from build123d import *

# Parameters (mm, degrees)
SKETCH1_W            = 20
SKETCH1_H            = 20
BOSS_EXTRUDE1_DEPTH  = 20
SKETCH2_W            = 45
SKETCH2_H            = 70
BOSS_EXTRUDE2_DEPTH  = 12
CUT_EXTRUDE1_DEPTH   = 5.8
FILLET1_R            = 3.6
FILLET2_R            = 10
SKETCH5_R            = 3.9
CUT_EXTRUDE2_DEPTH   = 53.490475326
CUT_EXTRUDE3_REACH   = 51.17
SKETCH6_R            = 1.75
SKETCH7_W            = 12
SKETCH7_H            = 45
CUT_EXTRUDE4_DEPTH   = 4.8
SKETCH9_W            = 12
SKETCH9_H            = 45
CUT_EXTRUDE5_DEPTH   = 23.8
SKETCH10_W           = 12.5
SKETCH10_H           = 41.4
CUT_EXTRUDE6_DEPTH   = 23.8
SKETCH11_W           = 20
SKETCH11_H           = 1.2
CUT_EXTRUDE7_DEPTH   = 23.8
BOSS_EXTRUDE3_START  = 20
SKETCH12_W           = 20
SKETCH12_H           = 20
SKETCH12_R           = 3.9
BOSS_EXTRUDE3_DEPTH  = 20
SKETCH13_W           = 20.2
SKETCH13_H           = 20.2
SKETCH13_R           = 3.9
BOSS_EXTRUDE4_DEPTH  = 40
SKETCH14_W           = 12
SKETCH14_H           = 20
BOSS_EXTRUDE5_DEPTH  = 0.1
SKETCH17_R           = 4.83091966
BOSS_EXTRUDE8_DEPTH  = 39
SKETCH18_W           = 20.2
SKETCH18_H           = 20.2
CUT_EXTRUDE8_DEPTH   = 40
FILLET4_R            = 4
SKETCH20_W           = 12
SKETCH20_H           = 20
BOSS_EXTRUDE9_DEPTH  = 8
SKETCH21_W           = 47.2
SKETCH21_H           = 20
BOSS_EXTRUDE11_DEPTH = 10
SKETCH23_W           = 20
SKETCH23_H           = 20
BOSS_EXTRUDE12_DEPTH = 30
SKETCH25_W           = 20
SKETCH25_H           = 40.2
BOSS_EXTRUDE13_DEPTH = 57.5
SKETCH26_W           = 20
SKETCH26_H           = 20.8
CUT_EXTRUDE9_DEPTH   = 40.9
SKETCH27_R           = 2.35
CUT_EXTRUDE10_DEPTH  = 10
SKETCH28_R           = 2.35
CUT_EXTRUDE11_DEPTH  = 140.85113514
CHAMFER1_SIZE        = 1
FILLET5_R            = 7


with BuildPart() as part:
    # Sketch1 → Boss-Extrude1 (new body)
    with BuildSketch(Plane(origin=(0, 0, 0), x_dir=(0, 0, -1), z_dir=(1, 0, 0))):
        Rectangle(SKETCH1_W, SKETCH1_H)
    extrude(amount=BOSS_EXTRUDE1_DEPTH)

    # Sketch2 → Boss-Extrude2 (add)
    with BuildSketch(Plane(origin=(20, 0, 0), x_dir=(0, 0, -1), z_dir=(1, 0, 0))):
        Rectangle(SKETCH2_W, SKETCH2_H)
    extrude(amount=BOSS_EXTRUDE2_DEPTH)

    # Sketch4 → Cut-Extrude1 (cut)
    with BuildSketch(Plane(origin=(32, 0, 0), x_dir=(0, 0, -1), z_dir=(1, 0, 0))):
        with BuildLine():
            Line((3.6, -28.55), (-3.6, -28.55))
            Line((-3.6, -28.55), (-3.6, -7.311805523))
            ThreePointArc((-3.6, -7.311805523), (0, 8.15), (3.6, -7.311805523))
            Line((3.6, -7.311805523), (3.6, -28.55))
        make_face()
    extrude(amount=-CUT_EXTRUDE1_DEPTH, mode=Mode.SUBTRACT)

    # Fillet1
    fillet1_edges = [part.edges().sort_by_distance(p)[0] for p in [
        (29.1, -28.55, 3.6),
        (29.1, -28.55, -3.6),
    ]]
    fillet(fillet1_edges, radius=FILLET1_R - 0.0001)  # a hair under: the kernel refuses the full size

    # Fillet2
    fillet2_edges = [part.edges().sort_by_distance(p)[0] for p in [
        (29.1, -7.311805523, 3.6),
        (29.1, -7.311805523, -3.6),
    ]]
    fillet(fillet2_edges, radius=FILLET2_R)

    # Sketch5 → Cut-Extrude2 (cut, through all)
    with BuildSketch(Plane.ZY):
        Circle(SKETCH5_R)
    extrude(amount=-CUT_EXTRUDE2_DEPTH, mode=Mode.SUBTRACT)

    # Sketch6 → Cut-Extrude3 (cut, up to next)
    with BuildSketch(Plane(origin=(26.2, 0, 0), x_dir=(0, 0, -1), z_dir=(1, 0, 0)), mode=Mode.PRIVATE) as cut_extrude3_sk1:
        with Locations((0, -20.6)):
            Circle(SKETCH6_R)
    cut_extrude3_tool1 = extrude(cut_extrude3_sk1.sketch, amount=-CUT_EXTRUDE3_REACH, mode=Mode.PRIVATE) & part.part
    # Sketch6 → Cut-Extrude3 (cut, up to next)
    with BuildSketch(Plane(origin=(26.2, 0, 0), x_dir=(0, 0, -1), z_dir=(1, 0, 0)), mode=Mode.PRIVATE) as cut_extrude3_sk2:
        with Locations((0, -9.35)):
            Circle(SKETCH6_R)
    cut_extrude3_tool2 = extrude(cut_extrude3_sk2.sketch, amount=-CUT_EXTRUDE3_REACH, mode=Mode.PRIVATE) & part.part
    add(cut_extrude3_tool1.solids().sort_by_distance((26.2, -20.6, 0))[0], mode=Mode.SUBTRACT)
    add(cut_extrude3_tool2.solids().sort_by_distance((26.2, -9.35, 0))[0], mode=Mode.SUBTRACT)

    # Sketch7 → Cut-Extrude4 (cut)
    with BuildSketch(Plane.XZ.offset(35)):
        with Locations((26, 0)):
            Rectangle(SKETCH7_W, SKETCH7_H)
    extrude(amount=-CUT_EXTRUDE4_DEPTH, mode=Mode.SUBTRACT)

    # Sketch9 → Cut-Extrude5 (cut)
    with BuildSketch(Plane(origin=(0, 35, 0), x_dir=(1, 0, 0), z_dir=(0, 1, 0))):
        with Locations((26, 0)):
            Rectangle(SKETCH9_W, SKETCH9_H)
    extrude(amount=-CUT_EXTRUDE5_DEPTH, mode=Mode.SUBTRACT)

    # Sketch10 → Cut-Extrude6 (cut)
    with BuildSketch(Plane.ZY.offset(-20)):
        with Locations((-16.25, -9.5)):
            Rectangle(SKETCH10_W, SKETCH10_H)
        with Locations((16.25, -9.5)):
            Rectangle(SKETCH10_W, SKETCH10_H)
    extrude(amount=-CUT_EXTRUDE6_DEPTH, mode=Mode.SUBTRACT)

    # Sketch11 → Cut-Extrude7 (cut)
    with BuildSketch(Plane.ZY.offset(-20)):
        with Locations((0, 10.6)):
            Rectangle(SKETCH11_W, SKETCH11_H)
    extrude(amount=-CUT_EXTRUDE7_DEPTH, mode=Mode.SUBTRACT)

    # Sketch12 → Boss-Extrude3 (add)
    with BuildSketch(Plane.ZY.offset(BOSS_EXTRUDE3_START)):
        Rectangle(SKETCH12_W, SKETCH12_H)
        Circle(SKETCH12_R, mode=Mode.SUBTRACT)
    extrude(amount=-BOSS_EXTRUDE3_DEPTH)

    # Sketch13 → Boss-Extrude4 (add)
    with BuildSketch(Plane.ZY.offset(20)):
        Rectangle(SKETCH13_W, SKETCH13_H)
        Circle(SKETCH13_R, mode=Mode.SUBTRACT)
    extrude(amount=-BOSS_EXTRUDE4_DEPTH)

    # Sketch14 → Boss-Extrude5 (add)
    with BuildSketch(Plane(origin=(0, 10, 0), x_dir=(1, 0, 0), z_dir=(0, 1, 0))):
        with Locations((26, 0)):
            Rectangle(SKETCH14_W, SKETCH14_H)
    extrude(amount=BOSS_EXTRUDE5_DEPTH)

    # Sketch17 → Boss-Extrude8 (add)
    with BuildSketch(Plane.ZY.offset(20)):
        Circle(SKETCH17_R)
    extrude(amount=-BOSS_EXTRUDE8_DEPTH)

    # Sketch18 → Cut-Extrude8 (cut)
    with BuildSketch(Plane.ZY.offset(20)):
        Rectangle(SKETCH18_W, SKETCH18_H)
    extrude(amount=-CUT_EXTRUDE8_DEPTH, mode=Mode.SUBTRACT)

    # Fillet4
    fillet4_edges = [part.edges().sort_by_distance(p)[0] for p in [
        (26, 10.1, -10),
        (26, 10.1, 10),
    ]]
    fillet(fillet4_edges, radius=FILLET4_R)

    # Sketch20 → Boss-Extrude9 (add)
    with BuildSketch(Plane.XZ.offset(30.2)):
        with Locations((26, 0)):
            Rectangle(SKETCH20_W, SKETCH20_H)
    extrude(amount=BOSS_EXTRUDE9_DEPTH)

    # Sketch21 → Boss-Extrude11 (add)
    with BuildSketch(Plane.XZ.offset(38.2)):
        with Locations((43.6, 0)):
            Rectangle(SKETCH21_W, SKETCH21_H)
    extrude(amount=BOSS_EXTRUDE11_DEPTH)

    # Sketch23 → Boss-Extrude12 (add)
    with BuildSketch(Plane.XZ.offset(48.2)):
        with Locations((57.2, 0)):
            Rectangle(SKETCH23_W, SKETCH23_H)
    extrude(amount=BOSS_EXTRUDE12_DEPTH)

    # Sketch25 → Boss-Extrude13 (add)
    with BuildSketch(Plane.XZ.offset(78.2)):
        with Locations((57.2, 0)):
            Rectangle(SKETCH25_W, SKETCH25_H)
    extrude(amount=BOSS_EXTRUDE13_DEPTH)

    # Sketch26 → Cut-Extrude9 (cut)
    with BuildSketch(Plane.XZ.offset(135.7)):
        with Locations((57.2, 0)):
            Rectangle(SKETCH26_W, SKETCH26_H)
    extrude(amount=-CUT_EXTRUDE9_DEPTH, mode=Mode.SUBTRACT)

    # Sketch27 → Cut-Extrude10 (cut)
    with BuildSketch(Plane(origin=(0, -135.7, 0), x_dir=(-1, 0, 0), z_dir=(0, -1, 0))):
        with Locations(Location((-57.2, 15.25, 0), (0, 0, 90))):
            Circle(SKETCH27_R)
        with Locations(Location((-57.2, -15.25, 0), (0, 0, 270))):
            Circle(SKETCH27_R)
    extrude(amount=-CUT_EXTRUDE10_DEPTH, mode=Mode.SUBTRACT)

    # Sketch28 → Cut-Extrude11 (cut, through all)
    with BuildSketch(Plane.ZY.offset(-47.2)):
        with Locations((4.9, -90.91)):
            Circle(SKETCH28_R)
        with Locations(Location((-4.9, -90.91, 0), (0, 0, 180))):
            Circle(SKETCH28_R)
    extrude(amount=-CUT_EXTRUDE11_DEPTH, mode=Mode.SUBTRACT)

    # Chamfer1
    chamfer1_edges = [part.edges().sort_by_distance(p)[0] for p in [
        (57.2, -135.7, -12.9),
        (57.2, -135.7, 12.9),
        (47.2, -90.91, 2.55),
        (47.2, -90.91, -2.55),
    ]]
    chamfer(chamfer1_edges, length=CHAMFER1_SIZE)

    # Fillet5
    fillet5_edges = [part.edges().sort_by_distance(p)[0] for p in [
        (32, -38.2, 0),
        (47.2, -48.2, 0),
    ]]
    fillet(fillet5_edges, radius=FILLET5_R)


solid = part.part
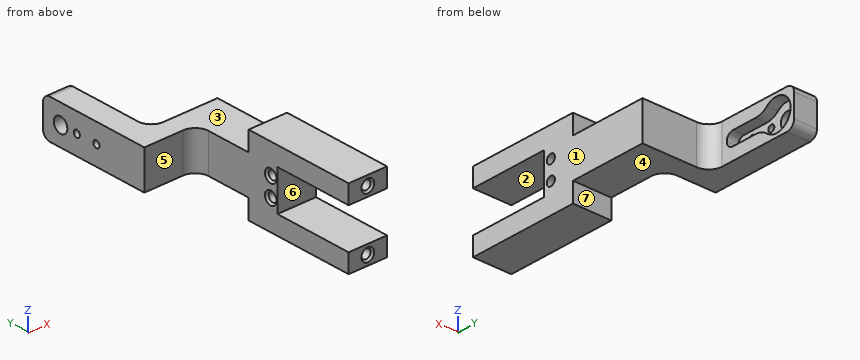
The model under review builds one solid part; all positions refer to its coordinate system, in mm. Face numbers are marked on the shaded views. A direction names the side the tool comes from. Give positions to 0.01 mm unless a question says otherwise; leave off trailing zeros. Order: outer loops, then holes, each group sorted by start corner. A loop starts at its lowest first (then second) coordinate and runs counter-clockwise, first axis right, second up. Notation, with made-up numbers: M 43.5,65 L 84.5,65 A16 ccw 84.5,95 Z; hole C -20,86.25 d2. An arc over 180 degrees is marked long. Use one line per item in the form item = value. Start each with the question number.
Item 1: To check wall thickness, follow line 1 along Y through (x, z) = (21.75, 0); line 2 along Y through (x, z) = (27.8, 0); line 3 along Z through (x, y) = (55.5, -92.5). State the ranges of each line that lie inside material, in increasing order. Write a range as from..to.
Item 2: We need section C-C on y = -15. Give the boundary of the cut face in (x, z), plus the area to 3 significant figures.
Item 3: For the marked faces 5, 6 and 7, list the 3-axis set-ups (+Z, -Z, +X, -X, +Y, -Y) from which the entire face can be reached by the end or side of a thin tool; tool diameter is ignored.
Item 4: We need section B-B on z = 15.25. Give the boundary of the cut face in (x, y).
Item 5: The part is to be moulded in two halves that separate along Z. For the marked faces 1, 2, 3 and 4, say which applies: pulls with the +Z half, pulls with the -Z half, needs draft (parallel to the pull), parting line crosses it, or undercut.
Item 6: Insertion check: pin 1 Ø10 at (x, z) = (31.5, 2) entering from -Y; pin 2 Ø2 at (y, z) = (-113, -14.5) entering from -X; pin 3 Ø1.5 at (x, y) = (53.5, -71) entering from +Z; pin 4 Ø6 at (x, z) = (36, 13.5) entering from -Y. Each pin has a flat end and moves straight along its axis. Give the tip position at first contact, or say it passes through.
Item 7: We need section D-D on x = 43.5. Give the boundary of the cut face in (y, z).
Completed:
q1.line_1 = -48.2..-22.35, -18.85..-11.1, -7.6..-3.9, 3.9..10.1
q1.line_2 = -48.2..-28.55, 8.15..10.1
q1.line_3 = -20.1..-6.63, -3.17..3.17, 6.63..20.1
q2.outline = M 20,-10 L 32,-10 L 32,-3.6 L 26.2,-3.6 L 26.2,3.6 L 32,3.6 L 32,10 L 20,10 Z
q2.area = 198 mm²
q3.face_5 = +Z, -Z, -X, -Y
q3.face_6 = +X, -X, -Y
q3.face_7 = -Z, +X, -X, +Y
q4.outline = M 47.2,-135.7 L 53.85,-135.7 L 54.85,-134.7 L 54.85,-125.7 L 59.55,-125.7 L 59.55,-134.7 L 60.55,-135.7 L 67.2,-135.7 L 67.2,-78.2 L 47.2,-78.2 Z
q5.face_1 = needs draft
q5.face_2 = undercut
q5.face_3 = pulls with the +Z half
q5.face_4 = pulls with the -Z half
q6.pin_1 = -48.2
q6.pin_2 = 47.2
q6.pin_3 = 10
q6.pin_4 = through
q7.outline = M -49.03,-10 L -38.2,-10 L -38.2,10 L -49.03,10 Z
